```python
from build123d import *

# Parameters (mm, degrees)
FILLET2_R        = 0.2
LPATTERN10_COUNT = 20
LPATTERN10_PITCH = 0.25


with BuildPart() as part:
    # Sketch1 → Revolve1 (revolve)
    with BuildSketch(Plane(origin=(0, 0, 0), x_dir=(1, 0, 0), z_dir=(0, 1, 0))):
        with BuildLine():
            Line((2.37, 1.5), (9.37, 1.5))
            Line((9.37, 1.5), (9.37, 0))
            Line((9.37, 0), (0, 0))
            ThreePointArc((0, 0), (0.224879408, 1.215980768), (0.869770135, 2.271109163))
            ThreePointArc((0.869770135, 2.271109163), (1.549177667, 2.754228297), (2.37, 2.9))
            Line((2.37, 2.9), (2.37, 1.5))
        make_face()
    revolve(axis=Axis((-13.629268293, 0, 0), (1, 0, 0)))

    # Fillet2
    fillet2_edges = [part.edges().sort_by_distance(p)[0] for p in [
        (2.37, 0, 1.5),
    ]]
    fillet(fillet2_edges, radius=FILLET2_R)

    # Sketch4 → Cut-Revolve1 (revolve, cut)
    with BuildSketch(Plane(origin=(0, 0, 0), x_dir=(1, 0, 0), z_dir=(0, 1, 0))):
        Polygon((10.103454633, 0), (10.103454633, 21), (-2.754355653, 21), (9.37, 0), align=None)
    revolve(axis=Axis((4.782773752, 0, 0), (1, 0, 0)), mode=Mode.SUBTRACT)

    # Sketch2 → Cut-Loft1 section 0
    with BuildSketch(Plane(origin=(0, 0, 0), x_dir=(0, 0, -1), z_dir=(1, 0, 0)), mode=Mode.PRIVATE) as cut_loft1_s0:
        Polygon((-0.4625, 0.4625), (-1.85, 0.4625), (-1.85, -0.4625), (-0.4625, -0.4625), (-0.4625, -1.85), (0.4625, -1.85), (0.4625, -0.4625), (1.85, -0.4625), (1.85, 0.4625), (0.4625, 0.4625), (0.4625, 1.85), (-0.4625, 1.85), align=None)
    loft([Vertex(2.62, 0, 0), cut_loft1_s0.sketch], mode=Mode.SUBTRACT)

    # Sketch6 → Cut-Revolve10 (revolve, cut)
    with BuildSketch(Plane.XY):
        Polygon((4.37, 1.7), (4.495, 1.7), (4.495, 1.5), (4.4325, 1.391746825), (4.37, 1.5), align=None)
    cut_revolve10 = revolve(axis=Axis((10.774329131, 0, 0), (-1, 0, 0)), mode=Mode.SUBTRACT)

    # LPattern10: Cut-Revolve10 ×20
    with Locations(*[(i * LPATTERN10_PITCH, 0, 0) for i in range(1, LPATTERN10_COUNT)]):
        add(cut_revolve10, mode=Mode.SUBTRACT)


solid = part.part
```
Check sheet for the modelled part. Datum: model origin and axes. Units: mm. A direction names the side the tool comes from. Coordinates: 2 decimals unless noted, no trailing zeros. Write each question's results on one line, items separated by ' | '. Start each with the question number.
1) Set-up check for faces 1 (the face through (1.04, 0.28, -0.62)), 2 (the face through (9.232, -0.092, -0.221)): record each of +Z, -Z, +X, -X, +Y, -Y from which the full face is reachable in a straight line by a thin tool's end or side.
2) Depth check by flat-ended pin: pin 1 (2 mm diameter, centred on x = 4, z = -1, fed in from -Y); pin 2 (1 mm diameter, centred on x = 3.5, z = 1.5, fed in from -Y); pin 3 (1 mm diameter, centred on x = 1.5, y = 2, fed in from +Z). Enter the tip coordinate at first touch or a pass-through.
3) Material ranges on line 1 along Y through (x, z) = (3, 0.8); line 2 along X through (y, z) = (0.7, 1.55); line 3 along Y through (x, z) = (2.75, 1.25), recorded low to high.
Checked values:
1) face 1: -X | face 2: +X
2) pin 1: y = -1.5 | pin 2: y = -1.12 | pin 3: z = 2.35
3) line 1: -1.27 to 1.27 | line 2: 0.46 to 2.37 | line 3: -0.83 to 0.83
